from build123d import *

# Parameters (mm, degrees)
F0_W           = 127
F0_H           = 127
F1_DEPTH       = 25.4
F2_R           = 25.4
F3_R           = 5.08
F5_D           = 12.7
F5_CSINK_D     = 19.05
F5_CSINK_ANGLE = 90


with BuildPart() as f1:
    # F0 (on Top) → F1 (new body)
    with BuildSketch(Plane.XY):
        Rectangle(F0_W, F0_H)
    extrude(amount=F1_DEPTH)

    # F2
    f2_edges = [f1.edges().sort_by_distance(p)[0] for p in [
        (63.5, -63.5, 12.7),
        (63.5, 63.5, 12.7),
        (-63.5, -63.5, 12.7),
        (-63.5, 63.5, 12.7),
    ]]
    fillet(f2_edges, radius=F2_R)

    # F3
    f3_edges = [f1.edges().sort_by_distance(p)[0] for p in [
        (0, -63.5, 25.4),
        (0, -63.5, 0),
    ]]
    fillet(f3_edges, radius=F3_R)

    # F5 (through all)
    with Locations(Plane.XY.offset(25.4)):
        with Locations((-38.1, -38.1), (-38.1, 38.1), (38.1, -38.1), (38.1, 38.1)):
            CounterSinkHole(F5_D / 2, F5_CSINK_D / 2, counter_sink_angle=F5_CSINK_ANGLE)


solid = f1.part
Read the model definition and answer for the solid it produces. Units are mm, in the model's axes. Coordinates: 2 decimals unless noted, no trailing zeros. Order: outer loops, then holes, each group sorted by start corner. A loop starts at its lowest first (then second) coordinate and runs counter-clockwise, first axis right, second up. Notation, with made-up numbers: (37.25, -0.5) - (51.25, -0.5) arc R29 cw to (51.25, 20.5) - close; hole circle Ø7 at (60.25, 2). An arc over 180 degrees is marked (long way). Use one line per item in the form item = value.
(1) Straight lines are drawn through the part: L1, parallel to X at y = -38.1, z = 11; L2, parallel to X at y = -41, z = 1.5. For each, find the intervals that lie inside material, in ascending order.
Computed values:
L1 = -63.5 to -44.45, -31.75 to 31.75, 44.45 to 63.5
L2 = -61.85 to -43.75, -32.45 to 32.45, 43.75 to 61.85
(2) For a pull along Y with two mould halves and no side action, classify faces 1 (the face through (34.6, 43.58, 22.38)), 2 (the face through (32.043, -36.193, 10.957)), 3 (the face through (-56.26, 55.86, 12.81)), 4 (the face through (61.972, 0.533, 1.449)) as pulls with the +Y half, pulls with the -Y half, needs draft (parallel to the pull), parting line crosses it, or undercut.
Computed values:
face_1 = undercut
face_2 = undercut
face_3 = pulls with the +Y half
face_4 = needs draft
(3) Given pin 1 Ø1.5 at (x, z) = (43.5, 16) entering from -Y; pin 2 Ø16.5 at (x, y) = (38.1, -38.1) entering from +Z (3 decimals), each flat-ended and moving along its own axis, determine where each tip first touches the part or whether it passes through.
Computed values:
pin_1 = -63.07
pin_2 = 24.125
(4) Section A-A, the plane z = 8.25 is taken. Give the vertices of the cut face in (x, y).
Computed values:
outline = (-63.5, -38.1) arc R25.4 ccw to (-38.1, -63.5) - (38.1, -63.5) arc R25.4 ccw to (63.5, -38.1) - (63.5, 38.1) arc R25.4 ccw to (38.1, 63.5) - (-38.1, 63.5) arc R25.4 ccw to (-63.5, 38.1) - close; hole circle Ø12.7 at (-38.1, -38.1); hole circle Ø12.7 at (-38.1, 38.1); hole circle Ø12.7 at (38.1, -38.1); hole circle Ø12.7 at (38.1, 38.1)
